```python
from build123d import *

# Parameters (mm, degrees)
SKETCH_W          = 67
SKETCH_H          = 48
SKETCH_R          = 3.15
SKETCH_R_2        = 5
PAD_DEPTH         = 2
FILLET_R          = 4
SKETCH001_R       = 21.5
PAD001_DEPTH      = 46
SKETCH002_W       = 36
SKETCH002_H       = 39
POCKET_DEPTH      = 33.501
POCKET_DEPTH_BACK = -33.501
SKETCH003_R       = 25
PAD002_DEPTH      = 35


with BuildPart() as part:
    # Sketch → Pad (new body)
    with BuildSketch(Plane.XY):
        Rectangle(SKETCH_W, SKETCH_H)
        with Locations((-27, 12)):
            Circle(SKETCH_R, mode=Mode.SUBTRACT)
        with Locations((27, -12)):
            Circle(SKETCH_R, mode=Mode.SUBTRACT)
        with Locations((27, 12)):
            Circle(SKETCH_R, mode=Mode.SUBTRACT)
        with Locations((-27, -12)):
            Circle(SKETCH_R, mode=Mode.SUBTRACT)
        Circle(SKETCH_R_2, mode=Mode.SUBTRACT)
    extrude(amount=PAD_DEPTH)

    # Fillet
    fillet_edges = [part.edges().sort_by_distance(p)[0] for p in [
        (-33.5, -24, 1),
        (33.5, -24, 1),
        (33.5, 24, 1),
        (-33.5, 24, 1),
    ]]
    fillet(fillet_edges, radius=FILLET_R)

    # Sketch001 (on Face5 of Fillet) → Pad001 (join)
    with BuildSketch(Plane.XY.offset(2)):
        Circle(SKETCH001_R)
    extrude(amount=PAD001_DEPTH)

    # Sketch002 → Pocket (cut, two sides)
    with BuildSketch(Plane.YZ) as pocket_sk:
        with Locations((0, 28.5)):
            Rectangle(SKETCH002_W, SKETCH002_H)
    extrude(amount=-POCKET_DEPTH, mode=Mode.SUBTRACT)
    extrude(pocket_sk.sketch, amount=-POCKET_DEPTH_BACK, mode=Mode.SUBTRACT)

    # Sketch003 (on Face21 of Pocket) → Pad002 (join)
    with BuildSketch(Plane.XZ.offset(-18)):
        with Locations((0, 39)):
            Circle(SKETCH003_R)
    extrude(amount=PAD002_DEPTH)


solid = part.part
```
Input: part model. Units: mm. Frame: model coordinates. A direction names the side the tool comes from. Coordinates: 2 decimals unless noted, no trailing zeros. Order: outer loops, then holes, each group sorted by start corner. A loop starts at its lowest first (then second) coordinate and runs counter-clockwise, first axis right, second up. Notation, with made-up numbers: (-8, 73.25) - (25, 73.25) arc R23 cw to (25, 102.25) - close; hole circle Ø6 at (-11, 19). An arc over 180 degrees is marked (long way). Put each result on its own line as item: value.
1. Reachability of faces 4 (the face through (0, 19, 48)), 5 (the face through (0, 0, 2)), 6 (the face through (0, -17, 39)), 7 (the face through (0, 0, 9)) from +Z, -Z, +X, -X, +Y, -Y: full face, straight path, thin tool, end or side. Return the list, or none.
Report:
face 4: +Z, +X, -X, +Y
face 5: -Z
face 6: +Z, +X, -X
face 7: +X, -X
2. Contact query for flat-ended pins moving along their axis: pin 1 Ø16 at (x, y) = (0, 0) entering from -Z; pin 2 Ø8 at (x, y) = (0, -0.5) entering from -Z; pin 3 Ø10 at (x, y) = (-27, 12) entering from +Z; pin 4 Ø24 at (x, y) = (-12, 12) entering from +Z. Output: stop coordinate, or through.
Report:
pin 1: stops at z = 0
pin 2: stops at z = 2
pin 3: stops at z = 50.87
pin 4: stops at z = 64
3. Draft query along Y for faces 1 (the face through (-32.359, 22.797, 1.014)), 2 (the face through (0, 18, 12)), 3 (the face through (0, 6, 0)). Return one class per face: pulls with the +Y half, pulls with the -Y half, needs draft (parallel to the pull), parting line crosses it, or undercut.
Report:
face 1: pulls with the +Y half
face 2: undercut
face 3: needs draft
4. Cut plane D-D on x = 0. Return the cut outline in (y, z).
Report:
outline: (-24, 0) - (-5, 0) - (-5, 2) - (5, 2) - (5, 0) - (24, 0) - (24, 2) - (21.5, 2) - (21.5, 48) - (18, 48) - (18, 64) - (-17, 64) - (-17, 14) - (18, 14) - (18, 9) - (-18, 9) - (-18, 48) - (-21.5, 48) - (-21.5, 2) - (-24, 2) - close
5. Cut plane B-B on y = 0. Return the cut outline in (x, z).
Report:
outline: (-33.5, 0) - (-5, 0) - (-5, 2) - (5, 2) - (5, 0) - (33.5, 0) - (33.5, 2) - (21.5, 2) - (21.5, 9) - (-21.5, 9) - (-21.5, 2) - (-33.5, 2) - close; circle Ø50 at (0, 39)
6. Cut plane A-A on x = -27. Return the cut outline in (y, z).
Report:
outline: (-24, 0) - (-15.15, 0) - (-15.15, 2) - (-24, 2) - close; (-8.85, 0) - (8.85, 0) - (8.85, 2) - (-8.85, 2) - close; (15.15, 0) - (24, 0) - (24, 2) - (15.15, 2) - close
7. Cut plane C-C on z = 38. Return the cut outline in (x, y).
Report:
outline: (-24.98, -17) - (24.98, -17) - (24.98, 18) - (11.76, 18) arc R21.5 ccw to (-11.76, 18) - (-24.98, 18) - close; (-11.76, -18) arc R21.5 ccw to (11.76, -18) - close
8. Line query: line 1 along Y through (x, z) = (-27, 1); line 2 along Y through (x, z) = (0, 1.3); line 3 along Y through (x, z) = (2, 49). Output: solid intervals per line, ascending.
Report:
line 1: y = -24 to -15.15, -8.85 to 8.85, 15.15 to 24
line 2: y = -24 to -5, 5 to 24
line 3: y = -17 to 18
